Can you work these out from the model? Positions are in its coordinate system, mm. A direction names the side the tool comes from. Coordinates: 2 decimals unless noted, no trailing zeros. Loops run counter-clockwise (first coordinate to the right, second up) from the corner with the lowest first, then second, coordinate; pieces in that order, holes last.
```python
from build123d import *

# Parameters (mm, degrees)
F0_W     = 60.0075
F0_H     = 86.36
F0_W_2   = 3.81
F0_H_2   = 3.81
F1_DEPTH = 6.35
F2_R     = 1.906977
F3_DEPTH = 86.361


with BuildPart() as f1:
    # F0 (on Front) → F1 (new body)
    with BuildSketch(Plane.XZ):
        with Locations((-30.00375, 43.18)):
            Rectangle(F0_W, F0_H)
        with Locations((-52.705, 36.195)):
            Rectangle(F0_W_2, F0_H_2, mode=Mode.SUBTRACT)
        with Locations((-52.705, 50.165)):
            Rectangle(F0_W_2, F0_H_2, mode=Mode.SUBTRACT)
    extrude(amount=F1_DEPTH)

    # F2 (on Top) → F3 (cut, through all)
    with BuildSketch(Plane.XY):
        with Locations((-3.81, -3.175)):
            Circle(F2_R)
    extrude(amount=F3_DEPTH, mode=Mode.SUBTRACT)


solid = f1.part
```
(1) If I drill on probe 1 along Z at (x, y) = (-53, -1.75); probe 2 along Y at (x, z) = (-3.81, 62.5); probe 3 along X at (y, z) = (-3, 5.5), over which ranges is the centre line in solid material (lowest first)?
Check values:
probe 1: z = 0 to 34.29, 38.1 to 48.26, 52.07 to 86.36
probe 2: y = -6.35 to -5.08, -1.27 to 0
probe 3: x = -60.01 to -5.71, -1.91 to 0
(2) I want a section at A-A on x = -3.81. Write out the boundary of the cut face in (y, z).
Check values:
outline: (-6.35, 0) - (-5.08, 0) - (-5.08, 86.36) - (-6.35, 86.36) - close; (-1.27, 0) - (0, 0) - (0, 86.36) - (-1.27, 86.36) - close
(3) I'm going to push a flat-ended pin straight in: pin 1 (3 mm diameter, centred on x = -3.81, y = -3.175, fed in from -Z). Where does the tip first touch, or does it pass through?
Check values:
pin 1: passes through
(4) I want a section at B-B on x = -52. Write out the boundary of the cut face in (y, z).
Check values:
outline: (-6.35, 0) - (0, 0) - (0, 34.29) - (-6.35, 34.29) - close; (-6.35, 38.1) - (0, 38.1) - (0, 48.26) - (-6.35, 48.26) - close; (-6.35, 52.07) - (0, 52.07) - (0, 86.36) - (-6.35, 86.36) - close
(5) If we mould it in two halves opening along X, with no side actions, what happens to faces 3 (the flat face through (-30, 0, 44)), 4 (the flat face through (-60.008, -3, 43)), 5 (the flat face through (-53, -3, 38.1))? For each: released by +X, released by -X, zero draft, split by the parting line, or undercut.
Check values:
face 3: zero draft
face 4: released by -X
face 5: undercut
(6) Which directions (+Z, -Z, +X, -X, +Y, -Y) give clear straight access to the entire face, cutting with the end or side of a thin tool? Please do faces 1 (the flat face through (-30, -3, 86.36)), 2 (the flat face through (-53, -3, 52.07)).
Check values:
face 1: +Z, +X, -X, +Y, -Y
face 2: +Y, -Y
